from build123d import *

# Parameters (mm, degrees)
SKETCH_1_R          = 4.6
EXTRUDE_1_DEPTH     = 9.8
SKETCH_2_R          = 4.6
SKETCH_2_R_2        = 4.4
CUT_EXTRUDE_1_DEPTH = 2
SKETCH_3_R          = 3.9
SKETCH_3_R_2        = 2.9
CUT_EXTRUDE_2_DEPTH = 4
SKETCH_4_R          = 2.4
CUT_EXTRUDE_3_DEPTH = 5
SKETCH_5_R          = 1.25
EXTRUDE_4_DEPTH     = 10
CHAMFER_1_SIZE      = 0.75
EXTRUDE_START       = 1
SKETCH_6_R          = 2.9
SKETCH_6_R_2        = 2.4
EXTRUDE_5_DEPTH     = 1
SKETCH_7_R          = 4
EXTRUDE_6_DEPTH     = 20
SKETCH_8_R          = 3.5
EXTRUDE_7_DEPTH     = 40


with BuildPart() as part:
    # 草图1 → 拉伸1 (new body)
    with BuildSketch(Plane(origin=(0, 0, 0), x_dir=(1, 0, 0), z_dir=(0, 1, 0))):
        with Locations(Location((0, 0, 0), (0, 0, 270))):
            Circle(SKETCH_1_R)
    extrude(amount=EXTRUDE_1_DEPTH)

    # 草图2 → 切除-拉伸1 (cut)
    with BuildSketch(Plane.XZ):
        with Locations(Location((0, 0, 0), (0, 0, 270))):
            Circle(SKETCH_2_R)
        with Locations(Location((0, 0, 0), (0, 0, 270))):
            Circle(SKETCH_2_R_2, mode=Mode.SUBTRACT)
    extrude(amount=-CUT_EXTRUDE_1_DEPTH, mode=Mode.SUBTRACT)

    # 草图3 → 切除-拉伸2 (cut)
    with BuildSketch(Plane.XZ):
        with Locations(Location((0, 0, 0), (0, 0, 270))):
            Circle(SKETCH_3_R)
        with Locations(Location((0, 0, 0), (0, 0, 270))):
            Circle(SKETCH_3_R_2, mode=Mode.SUBTRACT)
    extrude(amount=-CUT_EXTRUDE_2_DEPTH, mode=Mode.SUBTRACT)

    # 草图4 → 切除-拉伸3 (cut)
    with BuildSketch(Plane.XZ):
        with Locations(Location((0, 0, 0), (0, 0, 270))):
            Circle(SKETCH_4_R)
    extrude(amount=-CUT_EXTRUDE_3_DEPTH, mode=Mode.SUBTRACT)

    # 草图5 → 拉伸4 (add)
    with BuildSketch(Plane.XZ.offset(-5)):
        with Locations(Location((0, 0, 0), (0, 0, 270))):
            Circle(SKETCH_5_R)
    extrude(amount=EXTRUDE_4_DEPTH)

    # 倒角1
    chamfer_1_edges = [part.edges().sort_by_distance(p)[0] for p in [
        (0, -5, 1.25),
    ]]
    chamfer(chamfer_1_edges, length=CHAMFER_1_SIZE)

    # 草图6 → 拉伸5 (add)
    with BuildSketch(Plane.XZ.offset(EXTRUDE_START)):
        with Locations(Location((0, 0, 0), (0, 0, 270))):
            Circle(SKETCH_6_R)
        with Locations(Location((0, 0, 0), (0, 0, 270))):
            Circle(SKETCH_6_R_2, mode=Mode.SUBTRACT)
    extrude(amount=-EXTRUDE_5_DEPTH)

    # 草图7 → 拉伸6 (add)
    with BuildSketch(Plane(origin=(0, 9.8, 0), x_dir=(-1, 0, 0), z_dir=(0, 1, 0))):
        with Locations(Location((0, 0, 0), (0, 0, 90))):
            Circle(SKETCH_7_R)
    extrude(amount=EXTRUDE_6_DEPTH)

    # 草图8 → 拉伸7 (add)
    with BuildSketch(Plane(origin=(0, 29.8, 0), x_dir=(-1, 0, 0), z_dir=(0, 1, 0))):
        with Locations(Location((0, 0, 0), (0, 0, 90))):
            Circle(SKETCH_8_R)
    extrude(amount=EXTRUDE_7_DEPTH)


solid = part.part
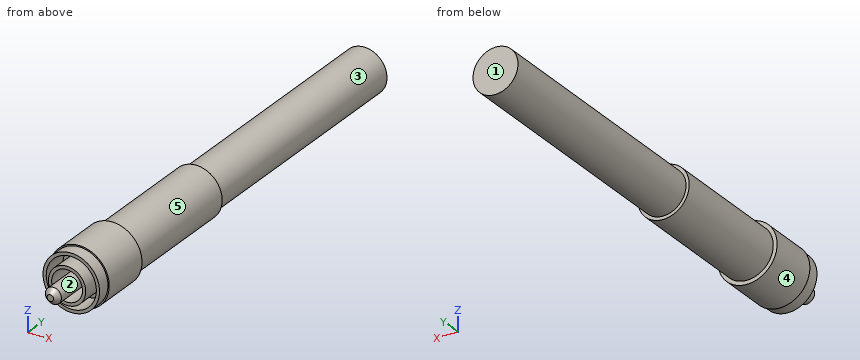
Check sheet for the modelled part. Datum: model origin and axes. Units: mm. Face numbers are marked on the shaded views. A direction names the side the tool comes from. Give positions to 0.01 mm unless a question says otherwise; leave off trailing zeros. Write each loop counter-clockwise with the first axis right and the second up, starting at its lowest first coordinate (ties: lowest second). Pieces come first, ordered by that corner, then holes. Notation, with made-up numbers: (16.25, 89) -> (45.25, 89) arc R13 ccw to (45.25, 100) -> close; hole circle Ø3 at (-34, 25). An arc over 180 degrees is marked (long way). One line per item, written item: value. Start each with the question number.
Item 1: Material ranges on probe 1 along X at (y, z) = (2.3, 0); probe 2 along X at (y, z) = (1.65, 0); probe 3 along Z at (x, y) = (-2.25, 6), recorded low to high. Write a range as from..to.
Item 2: Gauge pin test, flat ends, axial feed: pin 1 (2 mm diameter, centred on x = 2.5, z = 0, fed in from -Y); pin 2 (2.5 mm diameter, centred on x = -2, z = -1, fed in from -Y); pin 3 (1.4 mm diameter, centred on x = -1, z = 0.5, fed in from -Y); pin 4 (2 mm diameter, centred on x = -3.5, y = 13.5, fed in from +Z). Record the tip position at first contact, or that the pin passes through.
Item 3: Draft check along Z on the marked faces 1, 2 and 3. Enter one of: +Z half, -Z half, draft (parallel to the pull), parting line (faces both ways), or undercut.
Item 4: Tool access check on the marked faces 4 and 5. Record the directions out of +Z, -Z, +X, -X, +Y, -Y that give a thin tool (end or side, any length) a straight path to the whole face; none if there is none.
Item 5: Section check A-A on y = 63.5. Record the cut outline in (x, z), then the cut area to 3 significant figures.
Results list:
1. probe 1: -4.6..-3.9, -2.9..-2.4, -1.25..1.25, 2.4..2.9, 3.9..4.6
1. probe 2: -4.4..-3.9, -2.9..-2.4, -1.25..1.25, 2.4..2.9, 3.9..4.4
1. probe 3: -4.01..4.01
2. pin 1: y = -1
2. pin 2: y = -4.51
2. pin 3: y = -5
2. pin 4: z = 3.12
3. face 1: draft
3. face 2: undercut
3. face 3: parting line
4. face 4: +Y, -Y
4. face 5: +Y
5. outline: circle Ø7 at (0, 0)
5. area: 38.5 mm²
